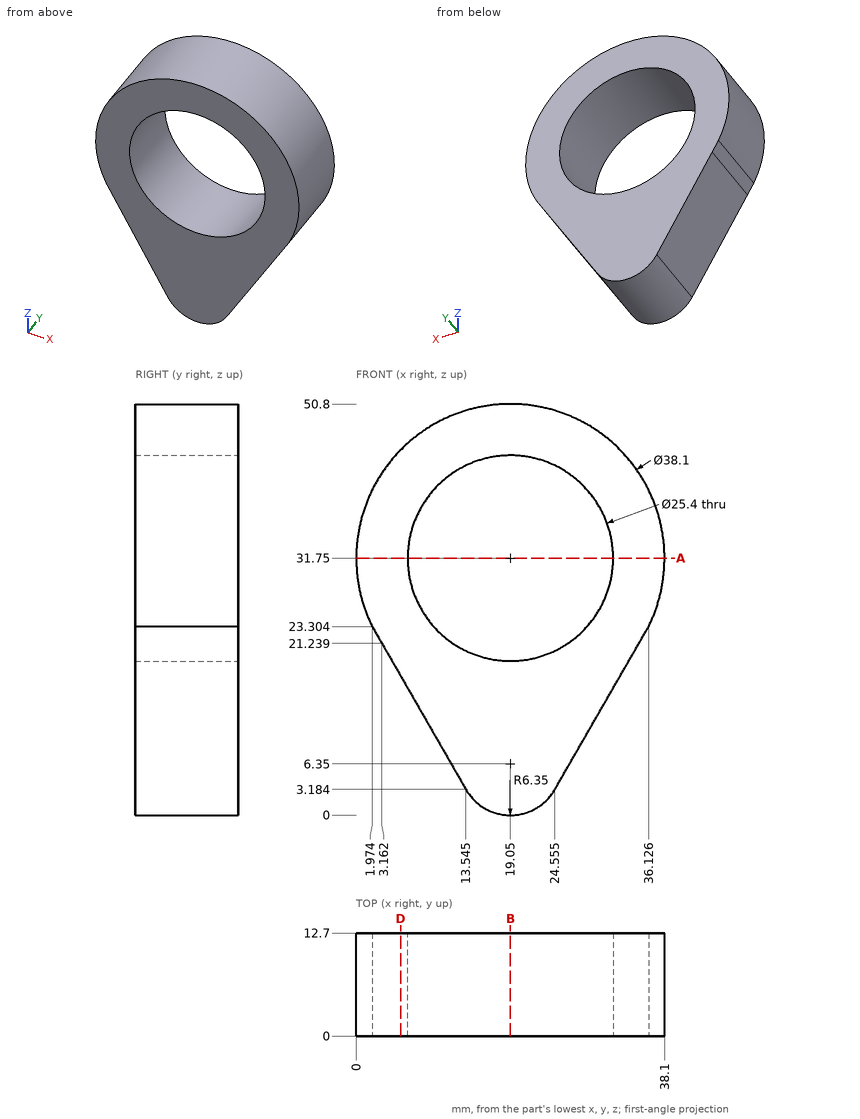
Geometry check sheet. Reference: drawing and pictorial views, mm from the part's lowest x, y, z. Coordinates: 2 decimals unless noted, no trailing zeros. Loops run counter-clockwise (first coordinate to the right, second up) from the corner with the lowest first, then second, coordinate; pieces in that order, holes last. Notation, with made-up numbers: (89, 45.5) - (130, 45.5) arc R10 cw to (130, 60.5) - close; hole circle Ø9 at (58.25, 44). An arc over 180 degrees is marked (long way). Return JSON: item names as keys, results as strings.
1. Thickness scan on L1, parallel to X at y = 2.25, z = 32.5 (1 decimal); L2, parallel to Z at x = 8, y = 9.75 (1 decimal); L3, parallel to X at y = 10.25, z = 36. Record the ranges inside material, lowest first.
Established:
{"L1": "x = 0 to 6.4, 31.7 to 38.1", "L2": "z = 12.8 to 25.5, 38 to 47.3", "L3": "x = 0.48 to 7.08, 31.02 to 37.62"}
2. Go/stop test with flat-tipped pins: pin 1 (3 mm diameter, centred on y = 4, z = 5.5, fed in from -X); pin 2 (1.5 mm diameter, centred on y = 1.5, z = 20, fed in from -X); pin 3 (2 mm diameter, centred on x = 7.5, y = 11, fed in from +Z); pin 4 (3 mm diameter, centred on x = 26, z = 45.5, fed in from -Y). Record where each tip stops, or that it passes through.
Established:
{"pin 1": "stops at x = 11.35", "pin 2": "stops at x = 3.44", "pin 3": "stops at z = 47.61", "pin 4": "stops at y = 0"}
3. Section check A-A, the plane z = 31.75. Record the boundary of the cut face in (x, y), then the cut area to 3 significant figures.
Established:
{"outline": "(0, 0) - (6.35, 0) - (6.35, 12.7) - (0, 12.7) - close; (31.75, 0) - (38.1, 0) - (38.1, 12.7) - (31.75, 12.7) - close", "area": "161 mm2"}
4. Section check D-D, the plane x = 5.5. Record the boundary of the cut face in (y, z).
Established:
{"outline": "(0, 17.17) - (12.7, 17.17) - (12.7, 45.14) - (0, 45.14) - close"}
5. Section check B-B, the plane x = 19.05. Record the boundary of the cut face in (y, z).
Established:
{"outline": "(0, 0) - (12.7, 0) - (12.7, 19.05) - (0, 19.05) - close; (0, 44.45) - (12.7, 44.45) - (12.7, 50.8) - (0, 50.8) - close"}
